The model under review builds one solid part; all positions refer to its coordinate system, in mm. A direction names the side the tool comes from. Round coordinates to 2 decimals unless told otherwise and drop trailing zeros. Loops run counter-clockwise (first coordinate to the right, second up) from the corner with the lowest first, then second, coordinate; pieces in that order, holes last. Notation, with made-up numbers: (68, 71) -> (109, 71) arc R16 cw to (109, 93) -> close; hole circle Ø11 at (48.5, -28). An arc over 180 degrees is marked (long way). Return JSON: item names as keys, results as strings. Group by question number.
```python
from build123d import *

# Parameters (mm, degrees)
F0_W      = 30
F0_H      = 81
F1_DEPTH  = 2.1
F2_W      = 30
F2_H      = 2.1
F3_DEPTH  = 51.2
F4_W      = 30
F4_H      = 2.1
F5_DEPTH  = 13.1
F6_W      = 30
F6_H      = 2.1
F7_DEPTH  = 16
F8_W      = 10.1
F8_H      = 10.2
F9_DEPTH  = 2.1
F11_DEPTH = 15.201
F13_DEPTH = 2.101
F14_R     = 2.1
F14_R_2   = 1.6
F15_DEPTH = 2.101
F16_W     = 2.1
F16_H     = 12.85
F17_DEPTH = 25
F18_R     = 1.1
F19_DEPTH = 25


with BuildPart() as f1:
    # F0 (on Front) → F1 (new body)
    with BuildSketch(Plane.XZ):
        Rectangle(F0_W, F0_H)
    extrude(amount=F1_DEPTH)

    # F2 (on face) → F3 (join)
    with BuildSketch(Plane.XZ.offset(2.1)):
        with Locations((0, -39.45)):
            Rectangle(F2_W, F2_H)
    extrude(amount=F3_DEPTH)

    # F4 (on face) → F5 (join)
    with BuildSketch(Plane.XY.offset(-38.4)):
        with Locations((0, -52.25)):
            Rectangle(F4_W, F4_H)
    extrude(amount=F5_DEPTH)

    # F6 (on face) → F7 (join)
    with BuildSketch(Plane.XZ.offset(53.3)):
        with Locations((0, -26.35)):
            Rectangle(F6_W, F6_H)
    extrude(amount=F7_DEPTH)

    # F8 (on face) → F9 (join)
    with BuildSketch(Plane.XY.offset(-25.3)):
        with Locations((-20.05, -64.2)):
            Rectangle(F8_W, F8_H)
        with Locations((20.05, -64.2)):
            Rectangle(F8_W, F8_H)
    extrude(amount=-F9_DEPTH)

    # F10 (on face) → F11 (cut, through all)
    with BuildSketch(Plane.XY.offset(-25.3)):
        with BuildLine():
            Line((-21.9, -63.2), (-21.9, -65.2))
            ThreePointArc((-21.9, -65.2), (-20.3, -66.8), (-18.7, -65.2))
            Line((-18.7, -65.2), (-18.7, -63.2))
            ThreePointArc((-18.7, -63.2), (-20.3, -61.6), (-21.9, -63.2))
        make_face()
        with BuildLine():
            Line((18.7, -63.2), (18.7, -65.2))
            ThreePointArc((18.7, -65.2), (20.3, -66.8), (21.9, -65.2))
            Line((21.9, -65.2), (21.9, -63.2))
            ThreePointArc((21.9, -63.2), (20.3, -61.6), (18.7, -63.2))
        make_face()
    extrude(amount=-F11_DEPTH, mode=Mode.SUBTRACT)

    # F12 (on face) → F13 (cut, through all)
    with BuildSketch(Plane.XY.offset(-38.4)):
        with BuildLine():
            Line((-15, -22.894339), (-9.15, -22.894339))
            ThreePointArc((-9.15, -22.894339), (-4.15, -17.894339), (-9.15, -12.894339))
            Line((-9.15, -12.894339), (-15, -12.894339))
            Line((-15, -12.894339), (-15, -22.894339))
        make_face()
    extrude(amount=-F13_DEPTH, mode=Mode.SUBTRACT)

    # F14 (on face) → F15 (cut, through all)
    with BuildSketch(Plane.XZ.offset(2.1)):
        with Locations((9, 35.6)):
            Circle(F14_R)
        with Locations((9, 11.6)):
            Circle(F14_R)
        with Locations((-9, 35.6)):
            Circle(F14_R)
        with Locations((-9, 11.6)):
            Circle(F14_R)
        with Locations((9, -9.2)):
            Circle(F14_R)
        with Locations((-9, -9.2)):
            Circle(F14_R)
        with Locations((6.05, -0.7)):
            Circle(F14_R_2)
        with Locations((-6.05, -0.7)):
            Circle(F14_R_2)
    extrude(amount=-F15_DEPTH, mode=Mode.SUBTRACT)

    # F16 (on face) → F17 (join)
    with BuildSketch(Plane(origin=(-15, 0, 0), x_dir=(0, -1, 0), z_dir=(-1, 0, 0))):
        with Locations((1.05, 34.075)):
            Rectangle(F16_W, F16_H)
    extrude(amount=F17_DEPTH)

    # F18 (on face) → F19 (cut)
    with BuildSketch(Plane.XZ.offset(2.1)):
        with Locations((-35.5, 37.425)):
            Circle(F18_R)
        with Locations((-35.5, 30.725)):
            Circle(F18_R)
    extrude(amount=-F19_DEPTH, mode=Mode.SUBTRACT)


solid = f1.part
```
1. For P1, Ø6.5, axis at x = 9, z = 35.6, coming from the -Y side; P2, Ø16.5, axis at y = -47.5, z = -35, coming from the -X side; P3, Ø2, axis at x = 14, y = -41.5, coming from the +Z side, all flat-tipped, find the tip position at first contact; note any pin that passes through.
2. We need section B-B, the plane x = 9. Write out the cut boundary in (y, z), then the cut area to 3 significant figures.
3. We need section A-A, the plane z = -30. Write out the cut boundary in (x, y).
4. We need section C-C, the plane x = -35.5. Write out the cut boundary in (y, z) (3 decimals).
5. Tool access review of faces 1 (the face through (-18.7, -64, -26)), 2 (the face through (0, -26, -38.4)), 3 (the face through (20, -59.1, -26)): name each direction out of +Z, -Z, +X, -X, +Y, -Y from which nothing blocks a thin tool from reaching the whole face with its end or side.
6. Wall thickness on line 1 (Z direction, x = -9, y = -0.65); line 2 (Z direction, x = -35.5, y = -1.55) (3 decimals); line 3 (Y direction, x = 12.5, z = -25.5): over which ranges is each line inside the solid? List them lowest first.
7. We need section D-D, the plane z = 10.5. Write out the cut boundary in (x, y).
8. Draft analysis for pull direction Y (two halves, no side actions). For faces 4 (the face through (-15, -1.6, -11.6)), 5 (the face through (-20, -59.1, -26)), 6 (the face through (-20.3, -66.8, -26.3)), 7 (the face through (-21.9, -64, -26)), state which applies: pulls with the +Y half, pulls with the -Y half, needs draft (parallel to the pull), parting line crosses it, or undercut.
Check sheet entries:
{
 "1": {"P1": "stops at y = -2.1", "P2": "stops at x = -15", "P3": "stops at z = -38.4"},
 "2": {"outline": "(-69.3, -27.4) -> (-53.3, -27.4) -> (-53.3, -40.5) -> (0, -40.5) -> (0, -11.3) -> (-2.1, -11.3) -> (-2.1, -38.4) -> (-51.2, -38.4) -> (-51.2, -25.3) -> (-69.3, -25.3) -> close; (-2.1, -7.1) -> (0, -7.1) -> (0, 9.5) -> (-2.1, 9.5) -> close; (-2.1, 13.7) -> (0, 13.7) -> (0, 33.5) -> (-2.1, 33.5) -> close; (-2.1, 37.7) -> (0, 37.7) -> (0, 40.5) -> (-2.1, 40.5) -> close", "area": "312 mm²"},
 "3": {"outline": "(-15, -53.3) -> (15, -53.3) -> (15, -51.2) -> (-15, -51.2) -> close; (-15, -2.1) -> (15, -2.1) -> (15, 0) -> (-15, 0) -> close"},
 "4": {"outline": "(-2.1, 27.65) -> (0, 27.65) -> (0, 29.625) -> (-2.1, 29.625) -> close; (-2.1, 31.825) -> (0, 31.825) -> (0, 36.325) -> (-2.1, 36.325) -> close; (-2.1, 38.525) -> (0, 38.525) -> (0, 40.5) -> (-2.1, 40.5) -> close"},
 "5": {"face 1": "+Z, -Z", "face 2": "+Z, +X, -X", "face 3": "+Z, -Z, +X, +Y"},
 "6": {"line 1": "z = -40.5 to -11.3, -7.1 to 9.5, 13.7 to 33.5, 37.7 to 40.5", "line 2": "z = 27.65 to 29.625, 31.825 to 36.325, 38.525 to 40.5", "line 3": "y = -69.3 to -51.2, -2.1 to 0"},
 "7": {"outline": "(-15, -2.1) -> (-10.79, -2.1) -> (-10.79, 0) -> (-15, 0) -> close; (-7.21, -2.1) -> (7.21, -2.1) -> (7.21, 0) -> (-7.21, 0) -> close; (10.79, -2.1) -> (15, -2.1) -> (15, 0) -> (10.79, 0) -> close"},
 "8": {"face 4": "needs draft", "face 5": "pulls with the +Y half", "face 6": "undercut", "face 7": "undercut"}
}
